from build123d import *

# Parameters (mm, degrees)
F1_DEPTH = 12.7
F2_DEPTH = 9.525
F3_DEPTH = 9.525
F4_D     = 10.3124


with BuildPart() as f1:
    # F0 (on Front) → F1 (new body)
    with BuildSketch(Plane.XZ):
        Polygon((-37.8326816705, -12.1775942421), (-29.7504506663, -20.2598252463), (-23.0152595659, -20.2598252463), (17.3958929789, -60.6709777911), (57.8070455237, -20.2598252463), (64.5422376145, -20.2598252463), (72.6244686187, -12.1775942421), (17.3958934741, 43.0509809025), align=None)
    extrude(amount=-F1_DEPTH)

    # F0 (on Front) → F2 (join)
    with BuildSketch(Plane.XZ):
        Polygon((111.0247183502, 64.0561261252), (-76.3002816498, 64.0561261252), (-76.3002816498, -20.2598252463), (-29.7504506663, -20.2598252463), (-37.8326816705, -12.1775942421), (17.3958934741, 43.0509809025), (72.6244686187, -12.1775942421), (64.5422376145, -20.2598252463), (111.0247183502, -20.2598252463), align=None)
    extrude(amount=F2_DEPTH)

    # F0 (on Front) → F3 (join)
    with BuildSketch(Plane.XZ):
        Polygon((-37.8326816705, -12.1775942421), (-29.7504506663, -20.2598252463), (-23.0152595659, -20.2598252463), (17.3958929789, -60.6709777911), (57.8070455237, -20.2598252463), (64.5422376145, -20.2598252463), (72.6244686187, -12.1775942421), (17.3958934741, 43.0509809025), align=None)
    extrude(amount=F3_DEPTH)

    # F4 (through all)
    with Locations(Plane(origin=(0, 0, 0), x_dir=(1, 0, 0), z_dir=(0, 1, 0))):
        with Locations((-58.8377816498, -48.1811261252), (-58.8377816498, -25.9561261252), (-58.8377816498, 12.1438738748), (93.5622183502, -48.1811261252), (93.5622183502, -25.9561261252), (93.5622183502, 12.1438738748)):
            Hole(F4_D / 2)


solid = f1.part
Input: part model. Units: mm. Frame: model coordinates. A direction names the side the tool comes from. Round coordinates to 2 decimals unless told otherwise and drop trailing zeros. Loops run counter-clockwise (first coordinate to the right, second up) from the corner with the lowest first, then second, coordinate; pieces in that order, holes last. Notation, with made-up numbers: M 46,3 L 99,3 A24 ccw 99,18 Z; hole C -30.75,-18 d3. An arc over 180 degrees is marked long. Answer as CSV lines item,"result". Start each with the question number.
(1) Section B-B, the plane z = 38. Output: boundary loops of the cut face in (x, y) (3 decimals).
(2) Section C-C, the plane y = 3.75. Output: boundary loops of the cut face in (x, z).
(3) First-contact query: pin 1 (12 mm diameter, centred on x = -58.84, z = 48.18, fed in from +Y); pin 2 (1.5 mm diameter, centred on y = -3.5, z = -31.5, fed in from +X); pin 3 (6.5 mm diameter, centred on x = 93, y = -1, fed in from -Z). Flat tips, straight axial feed; report the tip coordinate or a pass-through.
(4) Section A-A, the plane y = -5.25. Output: boundary loops of the cut face in (x, z), plus the area to 3 significant figures.
(5) Draft query along X for faces 1 (the cylindrical face through (88.8, -4.83, 50.16)), 2 (the flat face through (-5, 0, 32)), 3 (the cylindrical face through (-53.687, -4.829, -12.371)), 4 (the flat face through (37.319, 1.743, -40.748)). Return one class per face: released by +X, released by -X, zero draft, split by the parting line, or undercut.
(6) Section D-D, the plane x = 60.5. Output: boundary loops of the cut face in (y, z) (3 decimals), plus the area to 3 significant figures.
(7) Reachability of faces 5 (the flat face through (-33.85, 6.26, -16.16)), 6 (the flat face through (45.397, 6.261, 15.05)), 7 (the flat face through (84, -3, -20.26)), 8 (the flat face through (-9.832, 6.261, 15.823)), 9 (the flat face through (-50, -3, -20.26)) from +Z, -Z, +X, -X, +Y, -Y: full face, straight path, thin tool, end or side. Return the list, or none.
(8) Line query: line 1 (Y direction, x = 55, z = 53) (3 decimals); line 2 (X direction, y = -8.25, z = -8); line 3 (Z direction, x = 70, y = -8.5). Output: solid intervals per line, ascending. Write a range as [from, to].
Values found:
1,outline,"M -76.3,-9.525 L 111.025,-9.525 L 111.025,0 L 22.447,0 L 22.447,12.7 L 12.345,12.7 L 12.345,0 L -76.3,0 Z"
2,outline,"M -37.83,-12.18 L -29.75,-20.26 L -23.02,-20.26 L 17.4,-60.67 L 57.81,-20.26 L 64.54,-20.26 L 72.62,-12.18 L 17.4,43.05 Z"
3,pin 1,"stops at y = 0"
3,pin 2,"stops at x = 47.32"
3,pin 3,"stops at z = -20.26"
4,outline,"M -76.3,-20.26 L -23.02,-20.26 L 17.4,-60.67 L 57.81,-20.26 L 111.02,-20.26 L 111.02,64.06 L -76.3,64.06 Z; hole C -58.84,-12.14 d10.31; hole C -58.84,25.96 d10.31; hole C -58.84,48.18 d10.31; hole C 93.56,-12.14 d10.31; hole C 93.56,25.96 d10.31; hole C 93.56,48.18 d10.31"
4,area,"16,900 mm²"
5,face 1,"undercut"
5,face 2,"zero draft"
5,face 3,"undercut"
5,face 4,"released by +X"
6,outline,"M -9.525,-20.26 L 12.7,-20.26 L 12.7,-0.053 L 0,-0.053 L 0,64.056 L -9.525,64.056 Z"
6,area,"1,060 mm²"
7,face 5,"-Z, -X, +Y"
7,face 6,"+Z, +X, +Y"
7,face 7,"-Z, +X, +Y, -Y"
7,face 8,"+Z, -X, +Y"
7,face 9,"-Z, -X, +Y, -Y"
8,line 1,"y = [-9.525, 0]"
8,line 2,"x = [-76.3, -61.91], [-55.77, 90.49], [96.63, 111.02]"
8,line 3,"z = [-20.26, 64.06]"
